Check sheet for the modelled part. Datum: model origin and axes. Units: mm. Face numbers are marked on the shaded views. A direction names the side the tool comes from. Give positions to 0.01 mm unless a question says otherwise; leave off trailing zeros. Loops run counter-clockwise (first coordinate to the right, second up) from the corner with the lowest first, then second, coordinate; pieces in that order, holes last. Notation, with made-up numbers: (-31.75, -23.75) -> (11.25, -23.75) arc R24 cw to (11.25, 4.25) -> close; hole circle Ø9 at (3, -27.5). An arc over 180 degrees is marked (long way). Write each question's results on one line, items separated by ' | '. Start each with the question number.
Item 1: Access from +Z, -Z, +X, -X, +Y, -Y to the whole of each face (thin tool, end or side, straight path). Record for the marked faces 4, 5 and 6.
Item 2: Gauge pin test, flat ends, axial feed: pin 1 Ø0.8 at (y, z) = (-2, 11.5) entering from +X; pin 2 Ø15 at (x, y) = (21.5, 12) entering from +Z; pin 3 Ø4 at (x, y) = (1, 19.5) entering from +Z; pin 4 Ø1 at (x, z) = (41, 4.5) entering from -Y. Record the tip position at first contact, or that the pin passes through.
Item 3: Scan lines: line 1 along X through (y, z) = (0, 10.25); line 2 along X through (y, z) = (0, 5.5); line 3 along X through (y, z) = (23, 6). Record each from-to range of solid material in increasing order.
Item 4: Cross-section at A-A on z = 6.35. Enter the section's corners in (x, y), then the cut area to 3 significant figures.
Item 5: Cross-section at C-C on y = 0. Enter the section's corners in (x, z).
Item 6: Cross-section at B-B on x = 0. Enter the section's corners in (y, z), then the cut area to 3 significant figures.
Item 7: Cross-section at D-D on y = -18.5. Enter the section's corners in (x, z), then the cut area to 3 significant figures.
Item 8: Mould release check, pull along Y, two halves, no side actions. Record for the marked faces 1, 2 and 3: pulls with the +Y half, pulls with the -Y half, needs draft (parallel to the pull), parting line crosses it, or undercut.
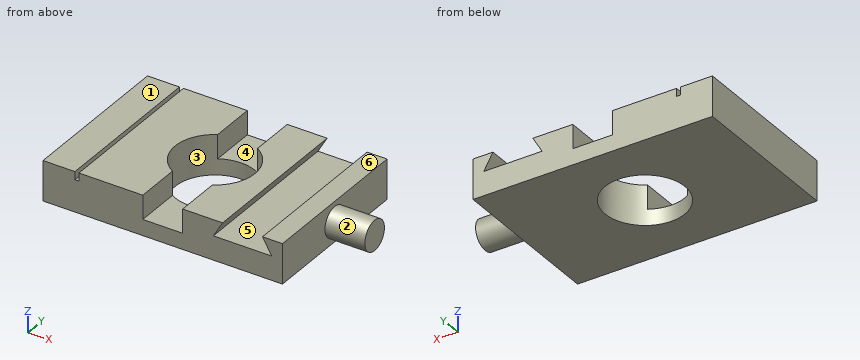
from build123d import *

# Parameters (mm, degrees)
F0_W     = 76.2
F0_H     = 50.8
F0_R     = 12.7
F1_DEPTH = 12.7
F3_DEPTH = 50.801
F5_DEPTH = 50.801
F6_R     = 4.7625
F7_DEPTH = 12.7


with BuildPart() as f1:
    # F0 (on Top) → F1 (new body)
    with BuildSketch(Plane.XY):
        Rectangle(F0_W, F0_H)
        Circle(F0_R, mode=Mode.SUBTRACT)
    extrude(amount=F1_DEPTH)

    # F2 (on face) → F3 (intersect, through all)
    with BuildSketch(Plane.XZ.offset(25.4)):
        Polygon((-27.94, 10.16), (-27.94, 12.7), (-38.1, 12.7), (-38.1, 0), (38.1, 0), (38.1, 12.7), (6.35, 12.7), (6.35, 5.08), (-6.35, 5.08), (-6.35, 12.7), (-26.67, 12.7), (-26.67, 10.16), align=None)
    extrude(amount=-F3_DEPTH, mode=Mode.INTERSECT)

    # F4 (on face) → F5 (cut, through all)
    with BuildSketch(Plane.XZ.offset(25.4)):
        Polygon((31.75, 12.7), (19.05, 12.7), (16.1170606325, 7.62), (34.6829393675, 7.62), align=None)
    extrude(amount=-F5_DEPTH, mode=Mode.SUBTRACT)

    # F6 (on face) → F7 (join)
    with BuildSketch(Plane.YZ.offset(38.1)):
        with Locations((0, 6.35)):
            Circle(F6_R)
    extrude(amount=F7_DEPTH)


solid = f1.part
Answer sheet:
1) face 4: +Z, +Y, -Y | face 5: +Y, -Y | face 6: +Z, +X, -X, +Y, -Y
2) pin 1: stops at x = 38.1 | pin 2: stops at z = 12.7 | pin 3: stops at z = 5.08 | pin 4: stops at y = -4.57
3) line 1: x = -38.1 to -27.94, -26.67 to -12.7, 12.7 to 17.64, 33.16 to 50.8 | line 2: x = -38.1 to -12.7, 12.7 to 50.8 | line 3: x = -38.1 to -6.35, 6.35 to 38.1
4) outline: (-38.1, -25.4) -> (-6.35, -25.4) -> (-6.35, -11) arc R12.7 cw to (-6.35, 11) -> (-6.35, 25.4) -> (-38.1, 25.4) -> close; (6.35, -25.4) -> (38.1, -25.4) -> (38.1, -4.76) -> (50.8, -4.76) -> (50.8, 4.76) -> (38.1, 4.76) -> (38.1, 25.4) -> (6.35, 25.4) -> (6.35, 11) arc R12.7 cw to (6.35, -11) -> close | area: 3,150 mm²
5) outline: (-38.1, 0) -> (-12.7, 0) -> (-12.7, 12.7) -> (-26.67, 12.7) -> (-26.67, 10.16) -> (-27.94, 10.16) -> (-27.94, 12.7) -> (-38.1, 12.7) -> close; (12.7, 0) -> (38.1, 0) -> (38.1, 1.59) -> (50.8, 1.59) -> (50.8, 11.11) -> (38.1, 11.11) -> (38.1, 12.7) -> (31.75, 12.7) -> (34.68, 7.62) -> (16.12, 7.62) -> (19.05, 12.7) -> (12.7, 12.7) -> close
6) outline: (-25.4, 0) -> (-12.7, 0) -> (-12.7, 5.08) -> (-25.4, 5.08) -> close; (12.7, 0) -> (25.4, 0) -> (25.4, 5.08) -> (12.7, 5.08) -> close | area: 129 mm²
7) outline: (-38.1, 0) -> (38.1, 0) -> (38.1, 12.7) -> (31.75, 12.7) -> (34.68, 7.62) -> (16.12, 7.62) -> (19.05, 12.7) -> (6.35, 12.7) -> (6.35, 5.08) -> (-6.35, 5.08) -> (-6.35, 12.7) -> (-26.67, 12.7) -> (-26.67, 10.16) -> (-27.94, 10.16) -> (-27.94, 12.7) -> (-38.1, 12.7) -> close | area: 788 mm²
8) face 1: needs draft | face 2: parting line crosses it | face 3: undercut
